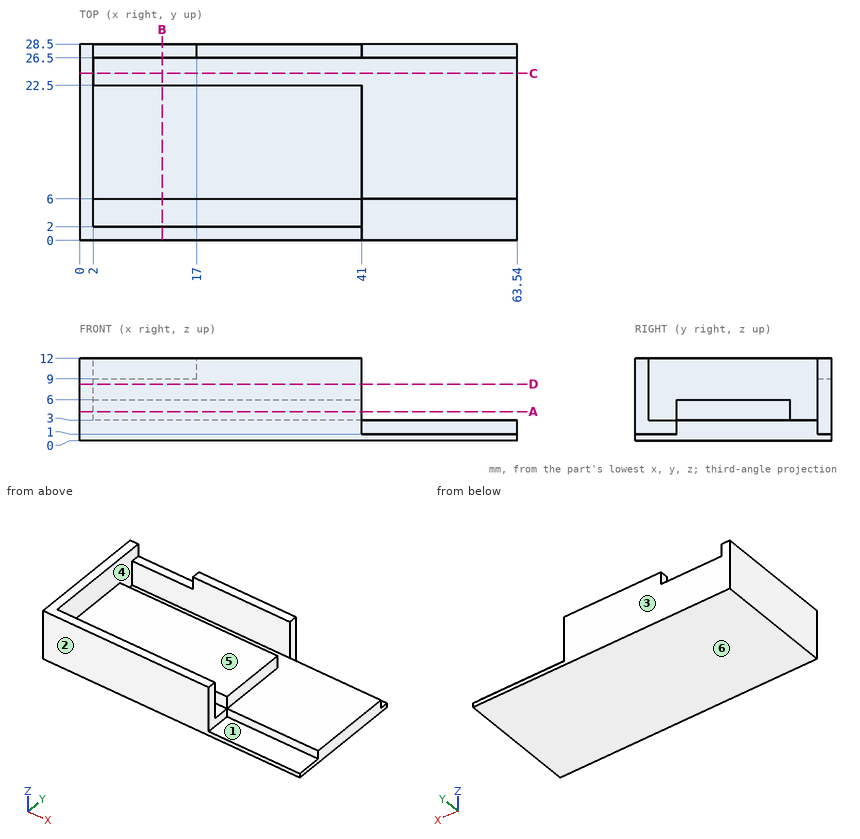
Design review of the part shown in the three views and the two pictorial views. Dimensions are in mm from the part's minimum x, y and z. A direction names the side the tool comes from. Coordinates: 2 decimals unless noted, no trailing zeros. Order: outer loops, then holes, each group sorted by start corner. A loop starts at its lowest first (then second) coordinate and runs counter-clockwise, first axis right, second up.
Item 1: Take a section at C-C, the plane y = 24.25. Write out the cut boundary in (x, z).
Item 2: Take a section at A-A, the plane z = 4.25. Write out the cut boundary in (x, y), then the cut area to 4 significant figures.
Item 3: For pin 1 Ø6.5 at (x, y) = (51, 1.5) entering from +Z; pin 2 Ø0.6 at (x, z) = (53.5, 2.5) entering from -Y; pin 3 Ø1.2 at (x, y) = (25, 4) entering from +Z, all flat-tipped, find the tip position at first contact; note any pin that passes through.
Item 4: Take a section at B-B, the plane x = 12. Write out the cut boundary in (y, z).
Item 5: The part is to be moulded in two halves that separate along Y. For the marked faces 1, 2, 3 and 4, say which applies: pulls with the +Y half, pulls with the -Y half, needs draft (parallel to the pull), parting line crosses it, or undercut.
Item 6: Take a section at D-D, the plane z = 8.25. Write out the cut boundary in (x, y), then the cut area to 3 significant figures.
Item 7: For the marked faces 5 and 6, list the 3-axis set-ups (+Z, -Z, +X, -X, +Y, -Y) from which the entire face can be reached by the end or side of a thin tool; tool diameter is ignored.
Item 8: For line 1 (Y direction, x = 7, z = 5.75); line 2 (Y direction, x = 37, z = 9); line 3 (Z direction, x = 4, y = 24.25), list the stretches that pass through material, from the lowest coordinate up.
The answers:
1. outline: (0, 0) - (63.54, 0) - (63.54, 3) - (2, 3) - (2, 12) - (0, 12) - close
2. outline: (0, 0) - (41, 0) - (41, 2) - (2, 2) - (2, 6) - (41, 6) - (41, 22.5) - (2, 22.5) - (2, 26.5) - (41, 26.5) - (41, 28.5) - (0, 28.5) - close
2. area: 856.5 mm2
3. pin 1: stops at z = 1
3. pin 2: stops at y = 6
3. pin 3: stops at z = 3
4. outline: (0, 0) - (28.5, 0) - (28.5, 9) - (26.5, 9) - (26.5, 3) - (22.5, 3) - (22.5, 6) - (6, 6) - (6, 3) - (2, 3) - (2, 12) - (0, 12) - close
5. face 1: needs draft
5. face 2: pulls with the -Y half
5. face 3: pulls with the +Y half
5. face 4: undercut
6. outline: (0, 0) - (41, 0) - (41, 2) - (2, 2) - (2, 26.5) - (41, 26.5) - (41, 28.5) - (0, 28.5) - close
6. area: 213 mm2
7. face 5: +Z, +X
7. face 6: -Z, +X, -X, +Y, -Y
8. line 1: y = 0 to 2, 6 to 22.5, 26.5 to 28.5
8. line 2: y = 0 to 2, 26.5 to 28.5
8. line 3: z = 0 to 3
